The drawing under review shows one solid part. Ordinate dimensions are in mm from its lowest x, y, z. Give positions to 0.01 mm unless a question says otherwise; leave off trailing zeros. Write each loop counter-clockwise with the first axis right and the second up, starting at its lowest first coordinate (ties: lowest second). Pieces come first, ordered by that corner, then holes. Notation, with made-up numbers: M 5.25,-14.5 L 50.25,-14.5 A8 ccw 50.25,0.5 Z; hole C 89,-17 d5. An arc over 180 degrees is marked long. Answer as a JSON object with one key per item and string values. Group by question number.
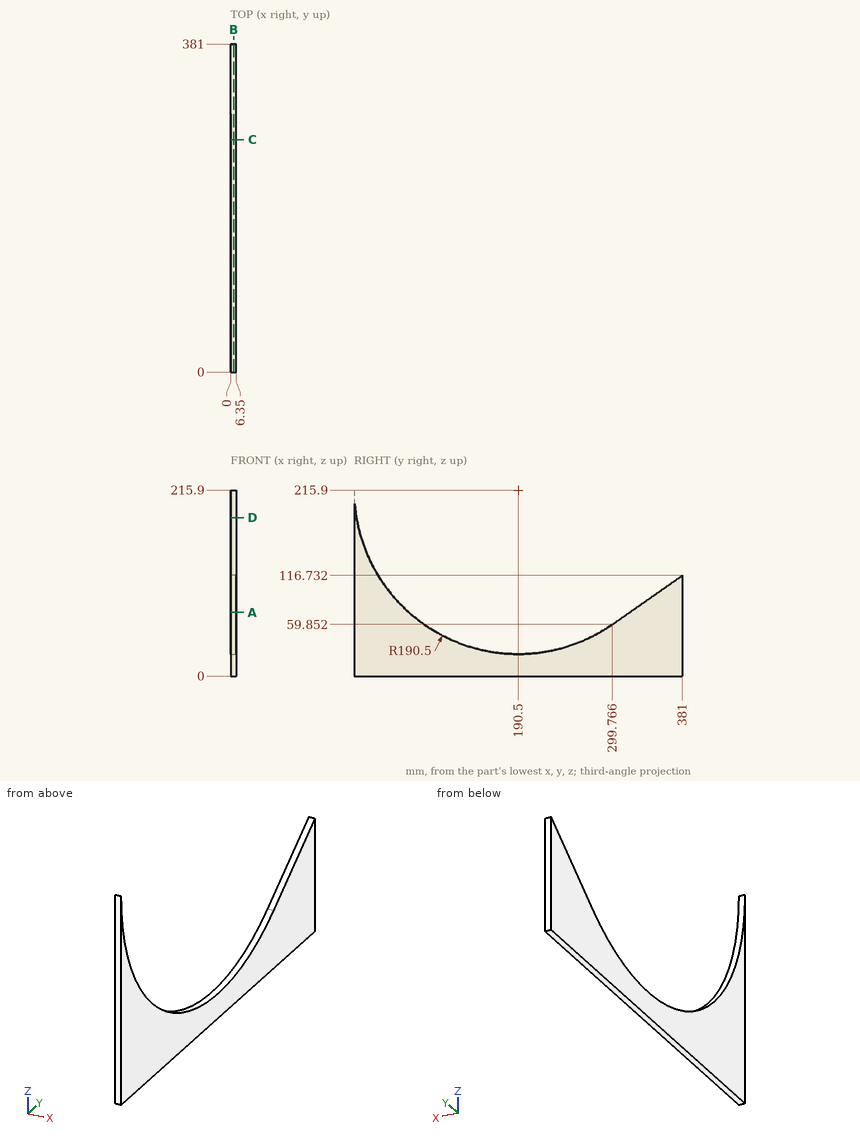
Item 1: To check wall thickness, follow probe 1 along Y at (x, z) = (2, 63) (1 decimal); probe 2 along Y at (x, z) = (1.75, 167.5); probe 3 along Y at (x, z) = (3.25, 81.5) (1 decimal). State the ranges of each line that lie inside material, in increasing order.
Item 2: Consider section D-D (z = 184). Give the boundary of the cut face in (x, y).
Item 3: Consider section A-A (z = 74). Give the boundary of the cut face in (x, y).
Item 4: Consider section C-C (y = 270). Give the boundary of the cut face in (x, z).
Item 5: Consider section B-B (x = 3.25). Give the boundary of the cut face in (y, z), plus the area to 3 significant figures.
Result set:
{
 "1": {"probe 1": "y = 0 to 76.9, 304.3 to 381", "probe 2": "y = 0 to 6.25", "probe 3": "y = 0 to 55.5, 330.7 to 381"},
 "2": {"outline": "M 0,0 L 6.35,0 L 6.35,2.69 L 0,2.69 Z"},
 "3": {"outline": "M 0,0 L 6.35,0 L 6.35,63.4 L 0,63.4 Z; M 0,319.97 L 6.35,319.97 L 6.35,381 L 0,381 Z"},
 "4": {"outline": "M 0,0 L 6.35,0 L 6.35,42.78 L 0,42.78 Z"},
 "5": {"outline": "M 0,0 L 381,0 L 381,116.73 L 299.77,59.85 A190.5 cw 0,215.9 Z", "area": "23,800 mm^2"}
}
